Autodesk Inventor part; units mm, degrees
ref_plane "YZ Plane" through (0, 0, 0) normal (1, 0, 0) x (0, 1, 0)
ref_plane "XZ Plane" through (0, 0, 0) normal (0, 1, 0) x (-1, 0, 0)
ref_plane "XY Plane" through (0, 0, 0) normal (0, 0, 1) x (1, 0, 0)
sketch "Boceto1" plane through (0, 0, 0) normal (0, 1, 0) x (-1, 0, 0)
  line L0 (17.5, -10) -> (-17.5, -10)
  line L1 (-17.5, -10) -> (-17.5, 10)
  line L2 (-17.5, 10) -> (17.5, 10)
  line L3 (17.5, 10) -> (17.5, 6.2798) construction
  line L4 (17.5, -10) -> (-17.5, 10) construction
  line L5 (-17.5, -10) -> (17.5, 10) construction
  line L6 (11.5, -6.25) -> (-11.5, -6.25)
  line L7 (-11.5, -6.25) -> (-11.5, 6.25)
  line L8 (-11.5, 6.25) -> (11.5, 6.25)
  line L9 (11.5, 6.25) -> (11.5, -6.25)
  line L10 (11.5, -6.25) -> (-11.5, 6.25) construction
  line L11 (-11.5, -6.25) -> (11.5, 6.25) construction
  arc A0 (36.6767, -6.9004) -> (36.6767, 6.9004) centre (35.5, 0) ccw
  line L12 (42.5, -10) -> (42.5, 4.9137) construction
  line L13 (37.6651, 3.75) -> (39.8301, 0)
  line L14 (39.8301, 0) -> (37.6651, -3.75)
  line L15 (37.6651, -3.75) -> (33.3349, -3.75)
  line L16 (33.3349, -3.75) -> (31.1699, 0)
  line L17 (31.1699, 0) -> (33.3349, 3.75)
  line L18 (33.3349, 3.75) -> (37.6651, 3.75)
  line L19 (28.5244, -2.7519) -> (26.9356, 0)
  line L20 (26.9356, 0) -> (28.5244, 2.7519)
  line L21 (17.5, -6.2798) -> (17.5, -10) construction
  line L22 (17.5, 6.2798) -> (17.5, -6.2798)
  line L23 (36.6767, -6.9004) -> (30, -6)
  line L24 (30, -6) -> (17.5, -10)
  line L25 (36.6767, 6.9004) -> (30, 6)
  line L26 (30, 6) -> (17.5, 10)
  line L27 (17.5, 6.2798) -> (28.5244, 2.7519)
  line L28 (17.5, -6.2798) -> (28.5244, -2.7519)
  point P0 (0, 0)
  point P1 (0, 0)
  point P2 (0, 0)
  point P3 (0, 0)
  point P4 (0, 0)
  point P5 (17.5, 10)
  dimension "d1" = 35
  dimension "d2" = 23
  dimension "d3" = 12.5
  dimension "d4" = 20
  dimension "d6" = 14
  dimension "d7" = 60
  dimension "d8" = 7.5
  dimension "d9" = 0
  dimension "d10" = 3.667
  dimension "d11" = 0
  dimension "d15" = 6
  dimension "d16" = 6
  dimension "d17" = 30
  dimension "d18" = 30
extrude "Extrusión1" add sketch "Boceto1" along normal blind 8
sketch "Boceto2" plane through (0, 8, 0) normal (0, 1, 0) x (1, 0, 0)
  circle A0 centre (-13.85, 0) radius 1
  circle A1 centre (13.85, 0) radius 1
  line L0 (0, 0) -> (0, -2.5102) construction
  dimension "d19" = 2
  dimension "d20" = 2
  dimension "d21" = 27.7
extrude "Extrusión2" cut sketch "Boceto2" against normal through all
sketch "Boceto3" plane through (0, 8, 0) normal (0, 1, 0) x (1, 0, 0)
  line L0 (11.5, 6.25) -> (11.5, -6.25)
  line L1 (11.5, 6.25) -> (11.5, -6.25)
  line L2 (11.5, 2.3) -> (13, 2.3)
  line L3 (13, 2.3) -> (13, -2.3)
  line L4 (13, -2.3) -> (11.5, -2.3)
  line L5 (11.5, -2.3) -> (11.5, 2.3)
  line L6 (0, 0) -> (1.0594, 0) construction
  point P0 (11.5, 2.3)
  point P1 (11.5, -2.3)
  dimension "d24" = 4.6
  dimension "d34" = 1.5
extrude "Extrusión3" cut sketch "Boceto3" against normal through all
chamfer "Chaflán1" distance 1.5 angle 45 8 edges at (0, 8, -10) (-23.75, 8, -8) (-33.3383, 8, -6.4502) (-42.5, 8, 0) (-33.3383, 8, 6.4502) (-23.75, 8, 8) (0, 8, 10) (17.5, 8, 0)
fillet "Empalme1" radius 6 1 edges at (-26.9356, 4, 0)
chamfer "Chaflán2" distance 1.5 angle 45 8 edges at (0, 0, 10) (17.5, 0, 0) (0, 0, -10) (-23.75, 0, -8) (-33.3383, 0, -6.4502) (-42.5, 0, 0) (-33.3383, 0, 6.4502) (-23.75, 0, 8)
properties part number "Tibia_V2"
Geometry check sheet. Reference: the model listing, model coordinates, mm. A direction names the side the tool comes from. Give positions to 0.01 mm unless a question says otherwise; leave off trailing zeros. Write each loop counter-clockwise with the first axis right and the second up, starting at its lowest first coordinate (ties: lowest second). Pieces come first, ordered by that corner, then holes.
1) Cross-section at B-B (x = 13.85). Record the boundary of the cut face in (y, z), plus the area to 4 significant figures.
Values follow:
outline: (0, -8.5) - (1.5, -10) - (6.5, -10) - (8, -8.5) - (8, -1) - (0, -1) - close; (0, 1) - (8, 1) - (8, 8.5) - (6.5, 10) - (1.5, 10) - (0, 8.5) - close
area: 139.5 mm2
2) Release check for a two-part mould opening along X. For faces 4 (the face through (17.5, 4, 0)), 5 (the face through (-35, 4, 3.75)), 6 (the face through (-0.2, 0.8, -9.3)), 7 (the face through (-36, 4, -3.75)) record: released by +X, released by -X, zero draft, split by the parting line, or undercut.
Values follow:
face 4: released by +X
face 5: undercut
face 6: zero draft
face 7: undercut
3) Cross-section at A-A (y = 5). Count the separate pieces of the cut face and the enclosed holes in it, plus the area to 3 significant figures.
Values follow:
separate pieces: 1
enclosed holes: 4
area: 600 mm2
4) Go/stop test with flat-tipped pins: pin 1 Ø3 at (x, z) = (-24.5, -7.5) entering from +Y; pin 2 Ø1.8 at (x, z) = (13.85, 0) entering from +Y; pin 3 Ø1.3 at (x, y) = (-36, 2.5) entering from +Z; pin 4 Ø2 at (x, y) = (-35, 2.5) entering from -Z. Record where each tip stops, or that it passes through.
Values follow:
pin 1: stops at y = 8
pin 2: passes through
pin 3: stops at z = 6.9
pin 4: stops at z = -6.81
5) Set-up check for faces 1 (the face through (0, 4, -10)), 2 (the face through (-22.94, 4.06, 4.54)), 3 (the face through (-23.84, 3.96, 7.97)): record each of +Z, -Z, +X, -X, +Y, -Y from which the full face is reachable in a straight line by a thin tool's end or side.
Values follow:
face 1: -Z, +X, -X, +Y, -Y
face 2: +Y, -Y
face 3: +Z, +Y, -Y
6) Thickness scan on line 1 (Z direction, x = 7.5, y = 6); line 2 (Z direction, x = -13.85, y = 2.5); line 3 (X direction, y = 5.5, z = -1.25). Record the ranges inside material, lowest first.
Values follow:
line 1: z = -10 to -6.25, 6.25 to 10
line 2: z = -10 to -1, 1 to 10
line 3: x = -42.39 to -39.11, -31.89 to -28, -17.5 to -11.5, 13 to 17.5
